```python
from build123d import *

# Parameters (mm, degrees)
CUT_EXTRUDE1_START = -2
CUT_EXTRUDE1_DEPTH = 2
SKETCH4_R          = 1.732050808
CUT_EXTRUDE2_DEPTH = 0.5
CUT_EXTRUDE2_TAPER = 45


with BuildPart() as part:
    # Sketch2 → Revolve1 (revolve)
    with BuildSketch(Plane(origin=(0, 0, 0), x_dir=(0, 0, -1), z_dir=(1, 0, 0))):
        Polygon((-9.8, 3.5), (-6.2, 3.5), (-6, 3.3), (-6, 2), (9.3, 2), (10, 1.3), (10, 0), (-10, 0), (-10, 3.3), align=None)
    revolve(axis=Axis((0, 0, -10), (0, 0, 1)))

    # Sketch3 → Cut-Extrude1 (cut)
    with BuildSketch(Plane.XY.offset(10).offset(CUT_EXTRUDE1_START)):
        Polygon((0, 1.732050808), (-1.5, 0.866025404), (-1.5, -0.866025404), (0, -1.732050808), (1.5, -0.866025404), (1.5, 0.866025404), align=None)
    extrude(amount=CUT_EXTRUDE1_DEPTH, mode=Mode.SUBTRACT)

    # Sketch4 → Cut-Extrude2 (cut)
    with BuildSketch(Plane.XY.offset(10)):
        Circle(SKETCH4_R)
    extrude(amount=-CUT_EXTRUDE2_DEPTH, taper=CUT_EXTRUDE2_TAPER, mode=Mode.SUBTRACT)


solid = part.part
```
Can you work these out from the model? Positions are in its coordinate system, mm. A direction names the side the tool comes from. Give positions to 0.01 mm unless a question says otherwise; leave off trailing zeros. Loops run counter-clockwise (first coordinate to the right, second up) from the corner with the lowest first, then second, coordinate; pieces in that order, holes last. Notation, with made-up numbers: M 75.25,21 L 125.25,21 A18 cw 125.25,38 Z; hole C 83.25,-35.75 d10. An arc over 180 degrees is marked long. One line per item, written item: value.
(1) Suppose I cut it at B-B on z = 6.75. List the corners of the cut face in (x, y) for me, plus the area to 3 significant figures.
Returned:
outline: C 0,0 d7
area: 38.5 mm^2
(2) Will these pins go through, and if not, where does the flat tip stop? pin 1 (1.5 mm diameter, centred on x = 1, z = -6, fed in from -Y); pin 2 (1.5 mm diameter, centred on x = 1.5, z = 3, fed in from +Y); pin 3 (2.5 mm diameter, centred on x = -0.5, y = -0.5, fed in from +Z); pin 4 (2 mm diameter, centred on y = -0.5, z = -7.5, fed in from -X).
Returned:
pin 1: y = -1.98
pin 2: y = 1.85
pin 3: z = 10
pin 4: x = -2
(3) I need wall thicknesses on line 1 (Z direction, x = 1.25, y = -2.5); line 2 (Y direction, x = 1, z = -8.5); line 3 (Y direction, x = -0.5, z = 1.25). Which ranges of each line are inside material? Lowest first, please.
Returned:
line 1: 6 to 10
line 2: -1.73 to 1.73
line 3: -1.94 to 1.94
(4) Suppose I cut it at C-C on z = -7. List the corners of the cut face in (x, y) for me.
Returned:
outline: C 0,0 d4
(5) We'd pull the mould along Y, two halves only. Please class faces 1 (the face through (-0.82, -1.39, 9.88)), 2 (the face through (-1.5, 0, 9)), 3 (the face through (2.2, 0, 6)), 4 (the face through (1.341, 3.233, 7.975)): released by +Y, released by -Y, zero draft, split by the parting line, or undercut.
Returned:
face 1: undercut
face 2: undercut
face 3: zero draft
face 4: split by the parting line
(6) Which directions (+Z, -Z, +X, -X, +Y, -Y) give clear straight access to the entire face, cutting with the end or side of a thin tool? Please do faces 5 (the face through (0.82, 1.39, 9.88)), 6 (the face through (0, 0, -10)), 7 (the face through (2, 0, -2)).
Returned:
face 5: +Z
face 6: -Z, +X, -X, +Y, -Y
face 7: -Z
(7) Suppose I cut it at A-A on y = 0. List the corners of the cut face in (x, z) for me, plus the area to 3 significant figures.
Returned:
outline: M -3.5,6.2 L -3.3,6 L -2,6 L -2,-9.3 L -1.3,-10 L 1.3,-10 L 2,-9.3 L 2,6 L 3.3,6 L 3.5,6.2 L 3.5,9.8 L 3.3,10 L 1.73,10 L 1.5,9.77 L 1.5,8 L -1.5,8 L -1.5,9.77 L -1.73,10 L -3.3,10 L -3.5,9.8 Z
area: 85.4 mm^2
